CAD build for the part. Positions are in the model's coordinates, mm. Face numbers are marked on the shaded views. Give positions to 0.01 mm unless a question says otherwise; leave off trailing zeros. Write each question's results on one line, items separated by ' | '. Start each with the question number.
```python
from build123d import *

# Parameters (mm, degrees)
BOSS_EXTRUDE1_DEPTH            = 5
CUT_EXTRUDE2_REACH             = 105.073
SKETCH2_R                      = 7.5
CUT_EXTRUDE2_DIRECTION_2_REACH = 105.073
CUT_EXTRUDE3_REACH             = 105.073
SKETCH3_W                      = 2.728932188
SKETCH3_H                      = 5
CUT_EXTRUDE3_DIRECTION_2_REACH = 105.073
FILLET1_R                      = 0.25


with BuildPart() as part:
    # Cam Profile Sketch → Boss-Extrude1 (new, symmetric)
    with BuildSketch(Plane.XY):
        with BuildLine():
            ThreePointArc((-95, 0), (-93.466662183, -11.64685703), (-88.97114317, -22.5))
            add(Edge.make_bspline(
                [(-24.019237886, -15), (-24.057726996, -15.066665093), (-24.135542603, -15.199984179), (-24.294210245, -15.468284804), (-24.486367794, -15.783992161), (-24.675050968, -16.085484944), (-24.8709034, -16.391428035), (-25.070085707, -16.695400658), (-25.371964938, -17.145687962), (-25.732401665, -17.664420975), (-26.25998012, -18.393991283), (-26.860454757, -19.180499871), (-27.42063933, -19.883348998), (-28.224273383, -20.853609638), (-28.932471155, -21.671343711), (-29.778521208, -22.611364699), (-30.768740875, -23.66727202), (-31.65162684, -24.579405423), (-32.935753353, -25.859926354), (-34.511627336, -27.360899541), (-36.401054833, -29.057445052), (-38.638036886, -30.906683495), (-40.962685031, -32.645088961), (-43.383053705, -34.248371754), (-45.959016936, -35.723391452), (-48.63808706, -37.003330144), (-51.412600635, -38.062115797), (-54.268660613, -38.876057715), (-57.122562395, -39.420836577), (-60.014975318, -39.698800922), (-62.92095712, -39.698748169), (-65.813153516, -39.414329857), (-68.733508438, -38.830455347), (-71.647577447, -37.928108287), (-74.516760762, -36.695099337), (-77.300501066, -35.127967674), (-79.581058345, -33.512324426), (-81.413170087, -31.971920034), (-82.710461133, -30.732394546), (-83.542718688, -29.87350859), (-84.214382827, -29.137329667), (-84.738529492, -28.536655846), (-85.245699359, -27.929262329), (-85.736176294, -27.316005605), (-86.328070579, -26.54398124), (-86.895689897, -25.761539987), (-87.388541821, -25.043964898), (-87.812126944, -24.397637278), (-88.0727685, -23.98897293), (-88.277415015, -23.661731501), (-88.47549914, -23.338928267), (-88.682364544, -22.994067163), (-88.846740598, -22.714364006), (-88.930106702, -22.571077248), (-88.97114317, -22.5)],
                knots=[0.066100625, 0.066100625, 0.066100625, 0.066100625, 0.066100625, 0.069918368, 0.07373611, 0.077553853, 0.081371596, 0.085189338, 0.089007081, 0.092824823, 0.104210915, 0.111779263, 0.126915961, 0.13448431, 0.142052658, 0.164824841, 0.172460326, 0.187731296, 0.203002265, 0.218273235, 0.248815158, 0.279357081, 0.309899022, 0.340440963, 0.3709829, 0.401524836, 0.434787958, 0.465329966, 0.495871896, 0.526413881, 0.556955827, 0.587497796, 0.618039752, 0.648581738, 0.682146995, 0.715712289, 0.749277564, 0.782842858, 0.799625499, 0.816408139, 0.82479946, 0.833190781, 0.841582102, 0.849973423, 0.858114254, 0.866255085, 0.882536748, 0.890677579, 0.894747995, 0.89881841, 0.902888826, 0.906959242, 0.911029657, 0.915100073, 0.915100073, 0.915100073, 0.915100073, 0.915100073], degree=4))
            ThreePointArc((-24.019237886, -15), (-20, 0), (-24.019237887, 15))
            add(Edge.make_bspline(
                [(-24.019237887, 15), (-24.068311179, 15.084997436), (-24.167781709, 15.254906705), (-24.372716614, 15.599220619), (-24.61865228, 15.997095978), (-24.863655112, 16.379697363), (-25.119128687, 16.767025959), (-25.379779341, 17.150163728), (-25.645266211, 17.528771772), (-25.945604472, 17.944852126), (-26.282522616, 18.396747851), (-26.657891266, 18.882728432), (-27.073733427, 19.401098012), (-27.605052795, 20.039628028), (-28.260315658, 20.790892876), (-29.137432462, 21.741660802), (-30.256936541, 22.871106034), (-31.513445882, 24.046837605), (-32.913450459, 25.258032474), (-34.702854921, 26.693691652), (-36.916722417, 28.304317086), (-39.592318083, 30.026272793), (-42.770642978, 31.770153659), (-46.070459158, 33.272672468), (-49.480743686, 34.50579862), (-53.151070656, 35.484877681), (-56.901056915, 36.10189034), (-60.695503134, 36.328853465), (-64.491489782, 36.145677899), (-68.078081084, 35.592442903), (-71.584996355, 34.657928649), (-74.969324852, 33.346617401), (-78.188701421, 31.670427503), (-81.216628819, 29.639247685), (-84.012954659, 27.273762593), (-86.22395529, 24.936788464), (-88.220215395, 22.396629412), (-89.728420053, 20.074270167), (-90.845118378, 18.05504037), (-91.819116647, 15.964820644), (-92.485619066, 14.320524673), (-92.985254722, 12.89744926), (-93.352941131, 11.710925817), (-93.616328574, 10.770894801), (-93.811723307, 10.014627811), (-94.03690859, 9.064875481), (-94.244035537, 8.074310703), (-94.430306675, 7.044765066), (-94.592927417, 5.974011134), (-94.710991165, 5.06120396), (-94.808756512, 4.141198889), (-94.886451771, 3.228074895), (-94.944318966, 2.297668795), (-94.977825799, 1.506610134), (-94.994478369, 0.807430389), (-94.999212886, 0.295654949), (-95, 0.0977871), (-95, 0)],
                knots=[0.066673701, 0.066673701, 0.066673701, 0.066673701, 0.066673701, 0.070604246, 0.074534791, 0.078465336, 0.082395881, 0.086326425, 0.09025697, 0.094187515, 0.09811806, 0.103762991, 0.109407922, 0.115052853, 0.120697784, 0.131987646, 0.143277509, 0.158999688, 0.174721868, 0.190444047, 0.206166227, 0.236936319, 0.267706411, 0.298476509, 0.329246606, 0.360016733, 0.390786859, 0.427383219, 0.45815328, 0.48892347, 0.519693606, 0.550463754, 0.581233829, 0.612004014, 0.642774165, 0.674103327, 0.705432525, 0.721097132, 0.752426343, 0.768090947, 0.783755547, 0.799420146, 0.81268856, 0.819322767, 0.825956974, 0.832591181, 0.839225388, 0.852493803, 0.860326099, 0.868158396, 0.875990693, 0.883822989, 0.891655286, 0.899487583, 0.90731988, 0.911236028, 0.915152176, 0.915152176, 0.915152176, 0.915152176, 0.915152176], degree=4))
        make_face()
    extrude(amount=BOSS_EXTRUDE1_DEPTH, both=True)

    # Sketch2 → Cut-Extrude2 (cut, up to next)
    with BuildSketch(Plane.XY, mode=Mode.PRIVATE) as cut_extrude2_sk1:
        with Locations((-50, 0)):
            Circle(SKETCH2_R)
    cut_extrude2_tool1 = extrude(cut_extrude2_sk1.sketch, amount=-CUT_EXTRUDE2_REACH, mode=Mode.PRIVATE) & part.part
    add(cut_extrude2_tool1.solids().sort_by_distance((-50, 0, 0))[0], mode=Mode.SUBTRACT)

    # Sketch2 → Cut-Extrude2 direction 2 (cut, up to next)
    with BuildSketch(Plane.XY, mode=Mode.PRIVATE) as cut_extrude2_direction_2_sk1:
        with Locations((-50, 0)):
            Circle(SKETCH2_R)
    cut_extrude2_direction_2_tool1 = extrude(cut_extrude2_direction_2_sk1.sketch, amount=CUT_EXTRUDE2_DIRECTION_2_REACH, mode=Mode.PRIVATE) & part.part
    add(cut_extrude2_direction_2_tool1.solids().sort_by_distance((-50, 0, 0))[0], mode=Mode.SUBTRACT)

    # Sketch3 → Cut-Extrude3 (cut, up to next)
    with BuildSketch(Plane.XY, mode=Mode.PRIVATE) as cut_extrude3_sk1:
        with Locations((-41.564466094, 0)):
            Rectangle(SKETCH3_W, SKETCH3_H)
    cut_extrude3_tool1 = extrude(cut_extrude3_sk1.sketch, amount=-CUT_EXTRUDE3_REACH, mode=Mode.PRIVATE) & part.part
    add(cut_extrude3_tool1.solids().sort_by_distance((-41.564466, 0, 0))[0], mode=Mode.SUBTRACT)

    # Sketch3 → Cut-Extrude3 direction 2 (cut, up to next)
    with BuildSketch(Plane.XY, mode=Mode.PRIVATE) as cut_extrude3_direction_2_sk1:
        with Locations((-41.564466094, 0)):
            Rectangle(SKETCH3_W, SKETCH3_H)
    cut_extrude3_direction_2_tool1 = extrude(cut_extrude3_direction_2_sk1.sketch, amount=CUT_EXTRUDE3_DIRECTION_2_REACH, mode=Mode.PRIVATE) & part.part
    add(cut_extrude3_direction_2_tool1.solids().sort_by_distance((-41.564466, 0, 0))[0], mode=Mode.SUBTRACT)

    # Fillet1
    fillet1_edges = [part.edges().sort_by_distance(p)[0] for p in [
        (-40.2, -2.5, 0),
        (-40.2, 2.5, 0),
    ]]
    fillet(fillet1_edges, radius=FILLET1_R)


solid = part.part
```
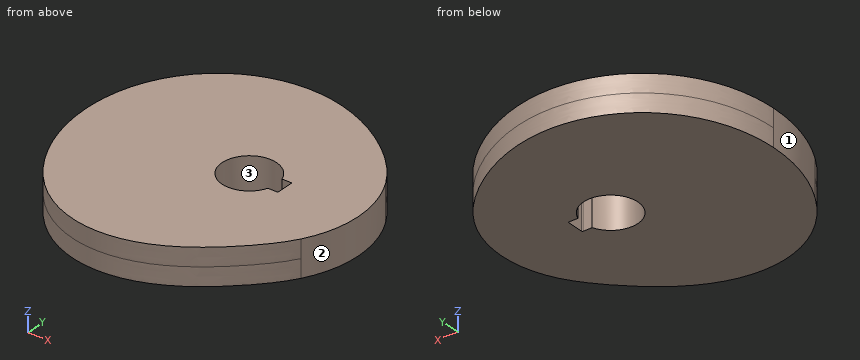
Q1. Wall check: L1, parallel to X at y = 0, z = 0; L2, parallel to Y at x = -50, z = -2.5; L3, parallel to X at y = -2, z = 0.5. Give the ranges that are in metal, low to high.
Q2. Drop flat-ended pins along their axis: pin 1 (6 mm diameter, centred on x = -29.5, z = -1, fed in from -Y); pin 2 (1.2 mm diameter, centred on x = -41.5, z = -2, fed in from -Y); pin 3 (17 mm diameter, centred on x = -50, y = 0, fed in from +Z); pin 4 (1 mm diameter, centred on y = -29.5, z = -2.5, fed in from -X). Give the stop position or say it passes through.
Q3. Mould opens along Y. For the marked faces 1, 2 and 3 say: pulls with the +Y half, pulls with the -Y half, needs draft (parallel to the pull), parting line crosses it, or undercut.
Answer block:
1) L1: x = -95 to -57.5, -40.2 to -20 | L2: y = -37.5 to -7.5, 7.5 to 34.6 | L3: x = -94.96 to -57.23, -40.2 to -20.07
2) pin 1: stops at y = -25.42 | pin 2: stops at y = -33.38 | pin 3: stops at z = 5 | pin 4: stops at x = -84.33
3) face 1: pulls with the -Y half | face 2: parting line crosses it | face 3: undercut
